Check sheet for the modelled part. Datum: model origin and axes. Units: mm. Face numbers are marked on the shaded views. A direction names the side the tool comes from. Round coordinates to 2 decimals unless told otherwise and drop trailing zeros. Write each loop counter-clockwise with the first axis right and the second up, starting at its lowest first coordinate (ties: lowest second). Pieces come first, ordered by that corner, then holes. Notation, with made-up numbers: (3, 20.25) -> (31, 20.25) arc R26 ccw to (31, 59.25) -> close; hole circle Ø2 at (57.25, 61). An arc over 180 degrees is marked (long way). One line per item, written item: value.
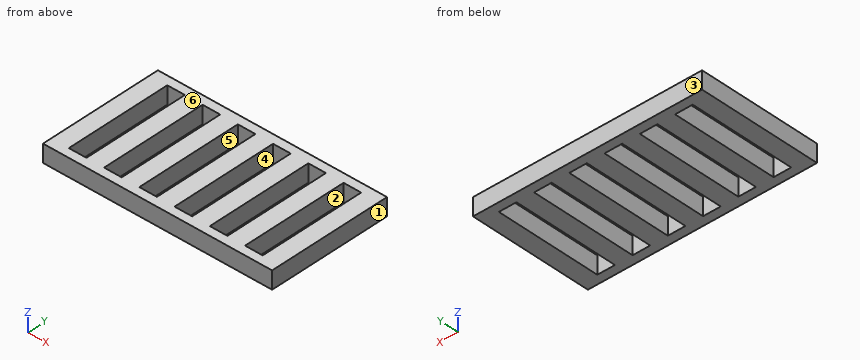
from build123d import *

# Parameters (mm, degrees)
F0_W     = 10
F0_H     = 60
F1_DEPTH = 10


with BuildPart() as f1:
    # F0 (on Top) → F1 (new body)
    with BuildSketch(Plane.XY):
        with Locations((-60, 0)):
            Rectangle(F0_W, F0_H)
        with Locations((-40, 0)):
            Rectangle(F0_W, F0_H)
        Polygon((65, 30), (65, 35), (-65, 35), (-65, 30), (-55, 30), (-45, 30), (-35, 30), (-25, 30), (-15, 30), (-5, 30), (5, 30), (15, 30), (25, 30), (35, 30), (45, 30), (55, 30), align=None)
        with Locations((-20, 0)):
            Rectangle(F0_W, F0_H)
        Rectangle(F0_W, F0_H)
        with Locations((20, 0)):
            Rectangle(F0_W, F0_H)
        with Locations((40, 0)):
            Rectangle(F0_W, F0_H)
        with Locations((60, 0)):
            Rectangle(F0_W, F0_H)
        Polygon((65, -35), (65, -30), (55, -30), (45, -30), (35, -30), (25, -30), (15, -30), (5, -30), (-5, -30), (-15, -30), (-25, -30), (-35, -30), (-45, -30), (-55, -30), (-65, -30), (-65, -35), align=None)
    extrude(amount=F1_DEPTH)


solid = f1.part
Item 1: Depth check by flat-ended pin: pin 1 (10 mm diameter, centred on x = -28, y = 3, fed in from -Z). Enter the tip coordinate at first touch or a pass-through.
Result set:
pin 1: z = 0
Item 2: Sectioned sample at C-C (z = 4.25). Enter the section's corners in (x, y).
Result set:
outline: (-65, -35) -> (65, -35) -> (65, 35) -> (-65, 35) -> close; hole (-55, -30) -> (-45, -30) -> (-45, 30) -> (-55, 30) -> close; hole (-35, -30) -> (-25, -30) -> (-25, 30) -> (-35, 30) -> close; hole (-15, -30) -> (-5, -30) -> (-5, 30) -> (-15, 30) -> close; hole (5, -30) -> (15, -30) -> (15, 30) -> (5, 30) -> close; hole (25, -30) -> (35, -30) -> (35, 30) -> (25, 30) -> close; hole (45, -30) -> (55, -30) -> (55, 30) -> (45, 30) -> close
Item 3: Tool access check on the marked faces 1 and 2. Record the directions out of +Z, -Z, +X, -X, +Y, -Y that give a thin tool (end or side, any length) a straight path to the whole face; none if there is none.
Result set:
face 1: +Z, -Z, +X, +Y, -Y
face 2: +Z, -Z
Item 4: Sectioned sample at B-B (y = 7). Enter the section's corners in (x, z), then the cut area to 3 significant figures.
Result set:
outline: (-65, 0) -> (-55, 0) -> (-55, 10) -> (-65, 10) -> close; (-45, 0) -> (-35, 0) -> (-35, 10) -> (-45, 10) -> close; (-25, 0) -> (-15, 0) -> (-15, 10) -> (-25, 10) -> close; (-5, 0) -> (5, 0) -> (5, 10) -> (-5, 10) -> close; (15, 0) -> (25, 0) -> (25, 10) -> (15, 10) -> close; (35, 0) -> (45, 0) -> (45, 10) -> (35, 10) -> close; (55, 0) -> (65, 0) -> (65, 10) -> (55, 10) -> close
area: 700 mm^2
Item 5: Release check for a two-part mould opening along Y. For the marked faces 3, 4, 5 and 6 record: pulls with the +Y half, pulls with the -Y half, needs draft (parallel to the pull), parting line crosses it, or undercut.
Result set:
face 3: pulls with the +Y half
face 4: undercut
face 5: undercut
face 6: needs draft
Item 6: Material ranges on line 1 along Y through (x, z) = (-33.5, 4), recorded low to high.
Result set:
line 1: -35 to -30, 30 to 35
Item 7: Sectioned sample at A-A (x = -9). Enter the section's corners in (y, z), then the cut area to 3 significant figures.
Result set:
outline: (-35, 0) -> (-30, 0) -> (-30, 10) -> (-35, 10) -> close; (30, 0) -> (35, 0) -> (35, 10) -> (30, 10) -> close
area: 100 mm^2
